Model file for the job. Use its own axes, mm. Face numbers are marked on the shaded views. A direction names the side the tool comes from. Round coordinates to 2 decimals unless told otherwise and drop trailing zeros. Loops run counter-clockwise (first coordinate to the right, second up) from the corner with the lowest first, then second, coordinate; pieces in that order, holes last. Notation, with made-up numbers: (-35, 37.25) -> (-4, 37.25) arc R30 ccw to (-4, 75.25) -> close; hole circle Ø3 at (26, 36.25). An arc over 180 degrees is marked (long way). Use a Markdown table: item, result.
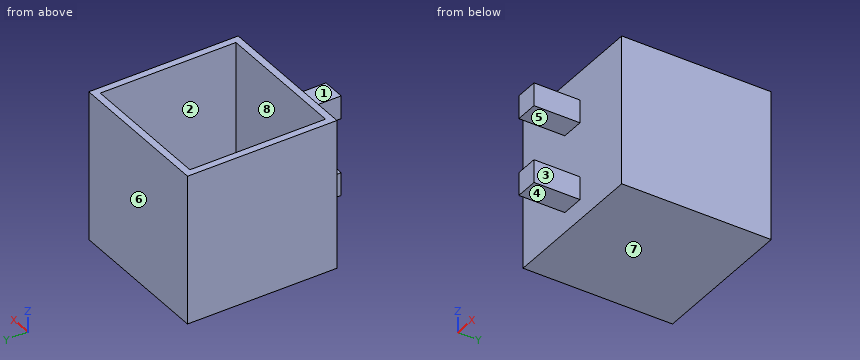
from build123d import *

# Parameters (mm, degrees)
F0_W     = 82.55
F0_H     = 82.55
F0_W_2   = 74.93
F0_H_2   = 74.93
F1_DEPTH = 82.55
F2_DEPTH = 3.81
F3_W     = 12.7
F3_H     = 12.7
F4_DEPTH = 25.4


with BuildPart() as f1:
    # F0 (on Top) → F1 (new body)
    with BuildSketch(Plane.XY):
        with Locations((62.48099, 6.929023)):
            Rectangle(F0_W, F0_H)
        with Locations((62.48099, 6.929023)):
            Rectangle(F0_W_2, F0_H_2, mode=Mode.SUBTRACT)
    extrude(amount=F1_DEPTH)

    # F0 (on Top) → F2 (join)
    with BuildSketch(Plane.XY):
        with Locations((62.48099, 6.929023)):
            Rectangle(F0_W_2, F0_H_2)
    extrude(amount=F2_DEPTH)

    # F3 (on face) → F4 (join)
    with BuildSketch(Plane.XZ.offset(34.345977)):
        with Locations((62.48099, 60.371522)):
            Rectangle(F3_W, F3_H)
        with Locations((62.48099, 17.477156)):
            Rectangle(F3_W, F3_H)
    extrude(amount=F4_DEPTH)


solid = f1.part
Q1. Band-saw the part on D-D, the plane y = -22.5. Give the cut face in (x, z), plus the area to 3 significant figures.
Results list:
| item | result |
|---|---|
| outline | (21.21, 0) -> (103.76, 0) -> (103.76, 82.55) -> (99.95, 82.55) -> (99.95, 3.81) -> (25.02, 3.81) -> (25.02, 82.55) -> (21.21, 82.55) -> close |
| area | 915 mm² |
Q2. Drill centre lines: L1, parallel to Y at x = 83.5, z = 53.5; L2, parallel to X at y = -17, z = 15.5; L3, parallel to Z at x = 53, y = -18.5. Where is each one in solid material? Low to high. Write a range as from..to.
Results list:
| item | result |
|---|---|
| L1 | y = -34.35..-30.54, 44.39..48.2 |
| L2 | x = 21.21..25.02, 99.95..103.76 |
| L3 | z = 0..3.81 |
Q3. Band-saw the part on C-C, the plane x = 95. Give the cut face in (y, z), plus the area to 3 significant figures.
Results list:
| item | result |
|---|---|
| outline | (-34.35, 0) -> (48.2, 0) -> (48.2, 82.55) -> (44.39, 82.55) -> (44.39, 3.81) -> (-30.54, 3.81) -> (-30.54, 82.55) -> (-34.35, 82.55) -> close |
| area | 915 mm² |
Q4. Band-saw the part on A-A, the plane y = -37.5. Give the cut face in (x, z).
Results list:
| item | result |
|---|---|
| outline | (56.13, 11.13) -> (68.83, 11.13) -> (68.83, 23.83) -> (56.13, 23.83) -> close; (56.13, 54.02) -> (68.83, 54.02) -> (68.83, 66.72) -> (56.13, 66.72) -> close |
Q5. Pull direction Y, two halves, no side cores. Call the marked faces 6, 7 and 8: released by +Y, released by -Y, zero draft, split by the parting line, or undercut.
Results list:
| item | result |
|---|---|
| face 6 | released by +Y |
| face 7 | zero draft |
| face 8 | undercut |
Q6. Flat gauge pins, fed straight in: pin 1 (8 mm diameter, centred on x = 47, z = 24.5, fed in from -Y); pin 2 (3 mm diameter, centred on x = 42, y = -22.5, fed in from -Z); pin 3 (10 mm diameter, centred on x = 60.5, y = -50, fed in from +Z); pin 4 (4 mm diameter, centred on x = 64.5, y = -45.5, fed in from -Z). Where does each tip first touch, or does it go through?
Results list:
| item | result |
|---|---|
| pin 1 | stops at y = -34.35 |
| pin 2 | stops at z = 0 |
| pin 3 | stops at z = 66.72 |
| pin 4 | stops at z = 11.13 |
Q7. Band-saw the part on B-B, the plane z = 48. Give the cut face in (x, y), plus the area to 3 significant figures.
Results list:
| item | result |
|---|---|
| outline | (21.21, -34.35) -> (103.76, -34.35) -> (103.76, 48.2) -> (21.21, 48.2) -> close; hole (25.02, -30.54) -> (99.95, -30.54) -> (99.95, 44.39) -> (25.02, 44.39) -> close |
| area | 1,200 mm² |
Q8. Tool access for the marked faces 1, 2, 3, 4 and 5: list every direction of +Z, -Z, +X, -X, +Y, -Y with a clear straight run to the whole face (end or side of a thin tool).
Results list:
| item | result |
|---|---|
| face 1 | +Z, +X, -X, -Y |
| face 2 | +Z |
| face 3 | +Z, -Z, +X, -Y |
| face 4 | -Z, +X, -X, -Y |
| face 5 | +X, -X, -Y |
